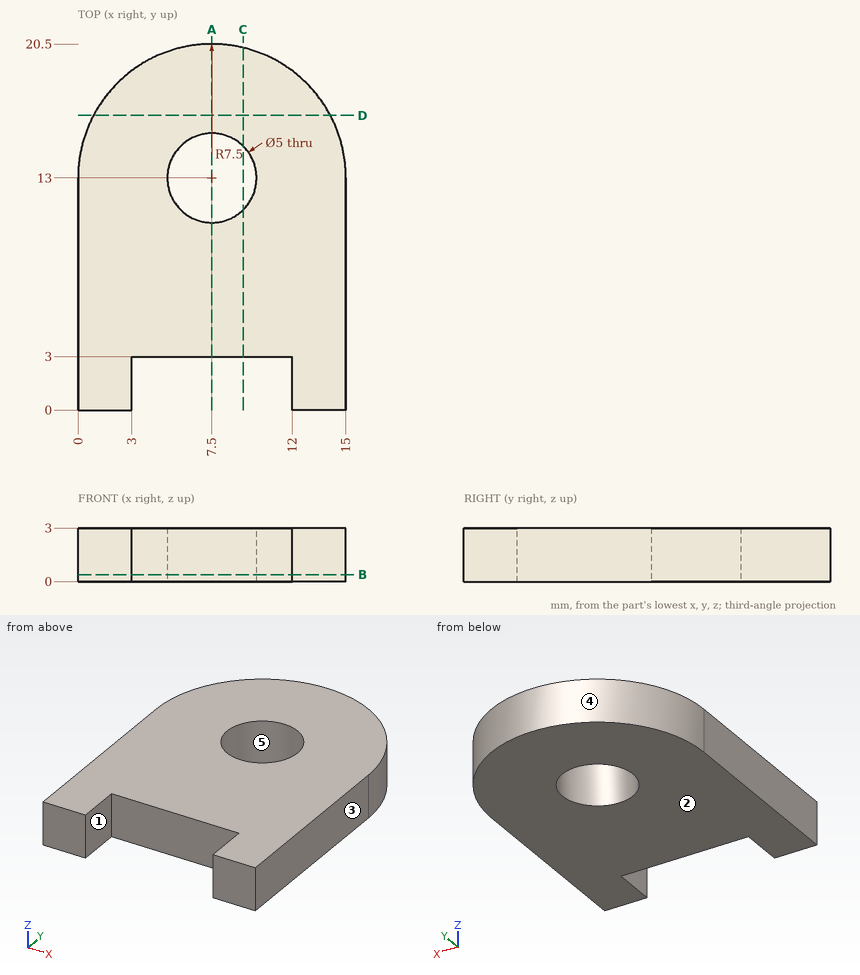
Source: three-view drawing plus pictorial views. Frame: mm from the lowest corner of the part. A direction names the side the tool comes from. Give positions to 0.01 mm unless a question says otherwise; leave off trailing zeros. Write each loop counter-clockwise with the first axis right and the second up, starting at its lowest first coordinate (ties: lowest second). Pieces come first, ordered by that corner, then holes. Notation, with made-up numbers: (-31, 56.5) -> (-18, 56.5) arc R24 cw to (-18, 87.5) -> close; hole circle Ø3 at (-15.5, 65). An arc over 180 degrees is marked (long way). Write item = value, one per line.
Q1. Line query: line 1 (Y direction, x = 7.5, z = 1.7); line 2 (X direction, y = 2.5, z = 0.4); line 3 (Y direction, x = 6.5, z = 1.35). Output: solid intervals per line, ascending. Write a range as from..to.
Here are the results:
line_1 = 3..10.5, 15.5..20.5
line_2 = 0..3, 12..15
line_3 = 3..10.71, 15.29..20.43
Q2. Cut plane D-D on y = 16.5. Return loops of the section in (x, z), then the cut area to 3 significant figures.
Here are the results:
outline = (0.87, 0) -> (14.13, 0) -> (14.13, 3) -> (0.87, 3) -> close
area = 39.8 mm²
Q3. Cut plane B-B on z = 0.4. Return loops of the section in (x, y), then the cut area to 3 significant figures.
Here are the results:
outline = (0, 0) -> (3, 0) -> (3, 3) -> (12, 3) -> (12, 0) -> (15, 0) -> (15, 13) arc R7.5 ccw to (0, 13) -> close; hole circle Ø5 at (7.5, 13)
area = 237 mm²
Q4. Cut plane C-C on x = 9.25. Return loops of the section in (y, z).
Here are the results:
outline = (3, 0) -> (11.21, 0) -> (11.21, 3) -> (3, 3) -> close; (14.79, 0) -> (20.29, 0) -> (20.29, 3) -> (14.79, 3) -> close
Q5. First-contact query: pin 1 (1.5 mm diameter, centred on x = 9.5, z = 1, fed in from +Y). Flat tip, straight axial feed; report the tip coordinate or a pass-through.
Here are the results:
pin_1 = 20.4
Q6. Mould query, pull axis X, two halves, no side actions, for the marked faces 3, 4 and 5. Classes: +X half, -X half, draft (parallel to the pull), parting line (faces both ways), or undercut.
Here are the results:
face_3 = +X half
face_4 = parting line
face_5 = undercut
Q7. Reachability of the marked faces 1 and 2 from +Z, -Z, +X, -X, +Y, -Y: full face, straight path, thin tool, end or side. Return the list, or none.
Here are the results:
face_1 = +Z, -Z, -Y
face_2 = -Z, +X, -X, +Y, -Y
Q8. Cut plane A-A on x = 7.5. Return loops of the section in (y, z), then the cut area to 3 significant figures.
Here are the results:
outline = (3, 0) -> (10.5, 0) -> (10.5, 3) -> (3, 3) -> close; (15.5, 0) -> (20.5, 0) -> (20.5, 3) -> (15.5, 3) -> close
area = 37.5 mm²
